Design review of the part built by this model. Coordinates are the model's own, in mm. A direction names the side the tool comes from. Round coordinates to 2 decimals unless told otherwise and drop trailing zeros. Loops run counter-clockwise (first coordinate to the right, second up) from the corner with the lowest first, then second, coordinate; pieces in that order, holes last. Notation, with made-up numbers: (-27, 53.5) -> (20, 53.5) arc R19 ccw to (20, 74.5) -> close; hole circle Ø11 at (-23.75, 37.25). An arc over 180 degrees is marked (long way). Answer as CSV lines item,"result". Start each with the question number.
(1) Take a section at A-A, the plane x = 0. Write out the cut boundary in (y, z), and give its area (3 significant figures).
(2) Draft analysis for pull direction Y (two halves, no side actions). For faces 3 (the face through (10.803, 24.45, 6.332)), 4 (the face through (-14.496, -2.507, 6.332)), 5 (the face through (1, 0, 1.27)), state which applies: +Y half, -Y half, draft (parallel to the pull), parting line (faces both ways), or undercut.
(3) To check wall thickness, follow line 1 (Z direction, x = 3.5, y = 0.5); line 2 (Y direction, x = 1, z = 2); line 3 (X direction, y = -12.5, z = 3.75). State the ranges of each line that lie inside material, in increasing order. Write a range as from..to.
(4) Machinability: for faces 1 (the face through (3, 0, 1)), 2 (the face through (16.953, -3.033, 6.332)), which of the approach directions +Z, -Z, +X, -X, +Y, -Y give a long, thin tool a straight path to every point of the face, cutting with its end or side? Answer none if there is none.
(5) For P1, Ø0.6, axis at x = 2.5, z = 0.5, coming from the +Y side; P2, Ø4, axis at x = 10.5, z = 4, coming from the +Y side (3 decimals); P3, Ø1, axis at x = 6, z = 4.5, coming from the +Y side; P4, Ø4, axis at x = 1.5, y = -4, coming from the -Z side, all flat-tipped, find the tip position at first contact; note any pin that passes through.
(6) Take a section at C-C, the plane z = 3.25. Write out the cut boundary in (x, y), and give its area (3 significant figures).
(7) Take a section at B-B, the plane y = -9.5. Write out the cut boundary in (x, z).
(8) Take a section at D-D, the plane x = -7.5. Write out the cut boundary in (y, z), and give its area (3 significant figures).
from build123d import *

# Parameters (mm, degrees)
F0_W     = 17.78
F0_H     = 31.9431498042
F1_DEPTH = 7.62
F2_SIZE2 = 7.62
F2_SIZE  = 5.08
F4_DEPTH = 1.27


with BuildPart() as f1:
    # F0 (on Top) → F1 (new body)
    with BuildSketch(Plane.XY):
        with Locations((1.2714529847, -2.1828604469)):
            Rectangle(F0_W, F0_H)
        Polygon((20.0711702637, 16.0299425669), (10.1614529847, 13.7887144552), (10.1614529847, -18.154435349), (13.9213964405, -21.5704601161), align=None)
        Polygon((-7.6185470153, -18.154435349), (-7.6185470153, 13.7887144552), (-17.5282642944, 16.0299425669), (-11.3784904712, -21.5704601161), align=None)
        Polygon((10.1614529847, -18.154435349), (-7.6185470153, -18.154435349), (-11.3784904712, -21.5704601161), (1.2714529847, -30.0696677594), (13.9213964405, -21.5704601161), align=None)
        Polygon((-17.5282642944, 16.0299425669), (-7.6185470153, 13.7887144552), (10.1614529847, 13.7887144552), (20.0711702637, 16.0299425669), (1.2714529847, 33.1100664022), align=None)
    extrude(amount=F1_DEPTH)

    # F2
    f2_edges = [f1.edges().sort_by_distance(p)[0] for p in [
        (-14.453377, -2.770259, 0),
        (-5.053519, -25.820064, 0),
        (7.596425, -25.820064, 0),
        (16.996283, -2.770259, 0),
        (10.671312, 24.570004, 0),
        (-8.128406, 24.570004, 0),
    ]]
    chamfer(f2_edges, length=F2_SIZE, length2=F2_SIZE2)

    # F3 (on face) → F4 (cut)
    with BuildSketch(Plane(origin=(0, 0, 0), x_dir=(1, 0, 0), z_dir=(0, 0, -1))):
        Polygon((1.3861381407, -1.0392206757), (1.3861381407, -15.0092206757), (4.0282764242, 0), (1.4882764242, 0), (1.3861381407, 13.9696266153), (-1.1537980354, -1.0572268218), align=None)
    extrude(amount=-F4_DEPTH, mode=Mode.SUBTRACT)


solid = f1.part
The answers:
1,outline,"(-29.22, 5.08) -> (-20.04, 0) -> (-5.77, 0) -> (-5.77, 1.27) -> (1.05, 1.27) -> (1.05, 0) -> (21.66, 0) -> (31.95, 5.08) -> (31.95, 7.62) -> (-29.22, 7.62) -> close"
1,area,"408 mm²"
2,face 3,"+Y half"
2,face 4,"-Y half"
2,face 5,"undercut"
3,line 1,"1.27..7.62"
3,line 2,"-24.32..26.62"
3,line 3,"-10.84..13.38"
4,face 1,"-Z"
4,face 2,"+Z, -Z, +X, -Y"
5,P1,"y = 23.38"
5,P2,"y = 26.255"
5,P3,"y = 28.75"
5,P4,"z = 0"
6,outline,"(-14.58, 15) -> (-8.86, -19.95) -> (1.27, -26.76) -> (11.4, -19.95) -> (17.12, 15) -> (1.27, 29.4) -> close"
6,area,"1,210 mm²"
7,outline,"(-13.35, 5.08) -> (-5.63, 0) -> (0.63, 0) -> (0.63, 1.27) -> (1.42, 1.27) -> (1.42, 0) -> (8.17, 0) -> (15.9, 5.08) -> (15.9, 7.62) -> (-13.35, 7.62) -> close"
8,outline,"(-24.18, 5.08) -> (-19.08, 2.26) -> (1.92, 0) -> (14.85, 0) -> (25.14, 5.08) -> (25.14, 7.62) -> (-24.18, 7.62) -> close"
8,area,"307 mm²"
